The model under review builds one solid part; all positions refer to its coordinate system, in mm. Round coordinates to 2 decimals unless told otherwise and drop trailing zeros. Order: outer loops, then holes, each group sorted by start corner. A loop starts at its lowest first (then second) coordinate and runs counter-clockwise, first axis right, second up.
from build123d import *

# Parameters (mm, degrees)
SKETCH2_R           = 2.50063
SKETCH2_R_2         = 3.5687
BOSS_EXTRUDE1_DEPTH = 4.7625


with BuildPart() as part:
    # Sketch2 → Boss-Extrude1 (new body)
    with BuildSketch(Plane.XY):
        with BuildLine():
            Line((20.204627806, -155.317842979), (66.653485088, -155.317842979))
            ThreePointArc((66.653485088, -155.317842979), (69.031331892, -154.332906584), (70.016268288, -151.95505978))
            Line((70.016268288, -151.95505978), (70.009462537, -134.779191139))
            ThreePointArc((70.009462537, -134.779191139), (69.330107736, -131.296239945), (67.723101309, -128.132381176))
            Line((67.723101309, -128.132381176), (58.368571144, -114.709141578))
            ThreePointArc((58.368571144, -114.709141578), (58.101227711, -114.164618042), (58.009428426, -113.56499209))
            Line((58.009428426, -113.56499209), (58.017340801, -89.273956224))
            ThreePointArc((58.017340801, -89.273956224), (58.109330305, -88.675027543), (58.376464494, -88.131136967))
            Line((58.376464494, -88.131136967), (67.309788153, -75.311850981))
            ThreePointArc((67.309788153, -75.311850981), (69.324850125, -71.208346949), (70.017816939, -66.689606297))
            Line((70.017816939, -66.689606297), (70.017970953, -58.209892985))
            ThreePointArc((70.017970953, -58.209892985), (67.203843889, -51.415989261), (60.409940165, -48.601862197))
            Line((60.409940165, -48.601862197), (20.204627806, -48.601862197))
            ThreePointArc((20.204627806, -48.601862197), (19.517944941, -48.72344088), (18.914748074, -49.073395554))
            Line((18.914748074, -49.073395554), (5.555020387, -60.347728592))
            ThreePointArc((5.555020387, -60.347728592), (4.951823521, -60.697683266), (4.265140655, -60.819261949))
            Line((4.265140655, -60.819261949), (-4.272604079, -60.819261949))
            ThreePointArc((-4.272604079, -60.819261949), (-4.959286944, -60.697683266), (-5.562483811, -60.347728592))
            Line((-5.562483811, -60.347728592), (-18.922211498, -49.073395554))
            ThreePointArc((-18.922211498, -49.073395554), (-19.525408364, -48.72344088), (-20.212091229, -48.601862197))
            Line((-20.212091229, -48.601862197), (-60.417403588, -48.601862197))
            ThreePointArc((-60.417403588, -48.601862197), (-67.211307313, -51.415989261), (-70.025434377, -58.209892985))
            Line((-70.025434377, -58.209892985), (-70.025280362, -66.689606297))
            ThreePointArc((-70.025280362, -66.689606297), (-69.332313549, -71.208346949), (-67.317251577, -75.311850981))
            Line((-67.317251577, -75.311850981), (-58.383927917, -88.131136967))
            ThreePointArc((-58.383927917, -88.131136967), (-58.116793729, -88.675027543), (-58.024804225, -89.273956224))
            Line((-58.024804225, -89.273956224), (-58.01689185, -113.56499209))
            ThreePointArc((-58.01689185, -113.56499209), (-58.108691135, -114.164618042), (-58.376034568, -114.709141578))
            Line((-58.376034568, -114.709141578), (-67.730564733, -128.132381176))
            ThreePointArc((-67.730564733, -128.132381176), (-69.337571159, -131.296239945), (-70.016925961, -134.779191139))
            Line((-70.016925961, -134.779191139), (-70.023731711, -151.95505978))
            ThreePointArc((-70.023731711, -151.95505978), (-69.038795316, -154.332906584), (-66.660948512, -155.317842979))
            Line((-66.660948512, -155.317842979), (-20.212091229, -155.317842979))
            ThreePointArc((-20.212091229, -155.317842979), (-19.525408364, -155.196264296), (-18.922211498, -154.846309622))
            Line((-18.922211498, -154.846309622), (-5.562483811, -143.571976584))
            ThreePointArc((-5.562483811, -143.571976584), (-4.959286944, -143.22202191), (-4.272604079, -143.100443227))
            Line((-4.272604079, -143.100443227), (4.265140655, -143.100443227))
            ThreePointArc((4.265140655, -143.100443227), (4.951823521, -143.22202191), (5.555020387, -143.571976584))
            Line((5.555020387, -143.571976584), (18.914748074, -154.846309622))
            ThreePointArc((18.914748074, -154.846309622), (19.517944941, -155.196264296), (20.204627806, -155.317842979))
        make_face()
        with Locations(Location((-56.926856711, -62.252536918, 0), (0, 0, 180))):
            Circle(SKETCH2_R, mode=Mode.SUBTRACT)
        with Locations(Location((-31.926856712, -62.252536918, 0), (0, 0, 180))):
            Circle(SKETCH2_R, mode=Mode.SUBTRACT)
        with Locations(Location((31.919393288, -62.252536918, 0), (0, 0, 180))):
            Circle(SKETCH2_R, mode=Mode.SUBTRACT)
        with Locations(Location((56.919393288, -62.252536918, 0), (0, 0, 180))):
            Circle(SKETCH2_R, mode=Mode.SUBTRACT)
        with Locations(Location((-39.920054199, -81.992843779, 0), (0, 0, 180))):
            Circle(SKETCH2_R, mode=Mode.SUBTRACT)
        with Locations(Location((-39.907032742, -91.992843779, 0), (0, 0, 180))):
            Circle(SKETCH2_R, mode=Mode.SUBTRACT)
        with Locations(Location((-39.920054199, -112.317382635, 0), (0, 0, 180))):
            Circle(SKETCH2_R, mode=Mode.SUBTRACT)
        with Locations(Location((-39.907032742, -132.632843676, 0), (0, 0, 180))):
            Circle(SKETCH2_R, mode=Mode.SUBTRACT)
        with Locations(Location((-39.920054199, -142.632843676, 0), (0, 0, 180))):
            Circle(SKETCH2_R, mode=Mode.SUBTRACT)
        with Locations(Location((10.02542097, -101.992843779, 0), (0, 0, 180))):
            Circle(SKETCH2_R, mode=Mode.SUBTRACT)
        with Locations(Location((-9.97457903, -101.992843779, 0), (0, 0, 180))):
            Circle(SKETCH2_R, mode=Mode.SUBTRACT)
        with Locations(Location((39.700429549, -91.992843779, 0), (0, 0, 180))):
            Circle(SKETCH2_R, mode=Mode.SUBTRACT)
        with Locations(Location((39.700429549, -132.632843676, 0), (0, 0, 180))):
            Circle(SKETCH2_R, mode=Mode.SUBTRACT)
        with Locations(Location((-56.895356292, -141.122536917, 0), (0, 0, 180))):
            Circle(SKETCH2_R_2, mode=Mode.SUBTRACT)
        with Locations(Location((39.700429549, -142.632843676, 0), (0, 0, 180))):
            Circle(SKETCH2_R_2, mode=Mode.SUBTRACT)
        with Locations(Location((39.700429549, -112.317382635, 0), (0, 0, 180))):
            Circle(SKETCH2_R_2, mode=Mode.SUBTRACT)
        with Locations(Location((39.700429549, -81.992843779, 0), (0, 0, 180))):
            Circle(SKETCH2_R_2, mode=Mode.SUBTRACT)
        with Locations(Location((56.887892868, -141.122536917, 0), (0, 0, 180))):
            Circle(SKETCH2_R_2, mode=Mode.SUBTRACT)
    extrude(amount=BOSS_EXTRUDE1_DEPTH)


solid = part.part
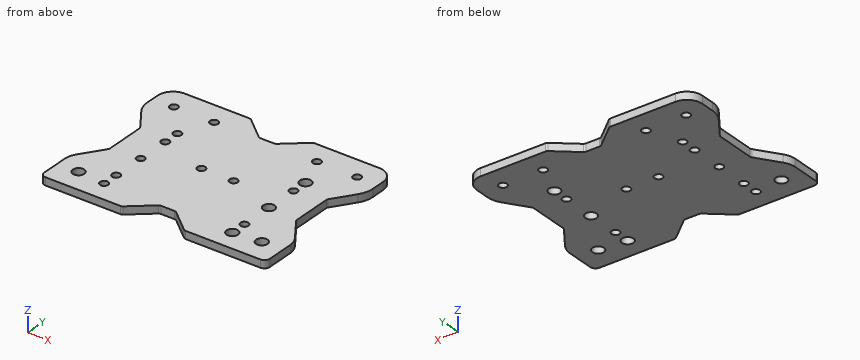
(1) Clearance check with flat-ended pins moving along their axes: P1, Ø4.5, axis at x = -9.97, y = -101.99, coming from the +Z side (3 decimals); P2, Ø1.4, axis at y = -100.5, z = 3, coming from the +X side; P3, Ø1.4, axis at y = -146, z = 3.5, coming from the +X side; P4, Ø1.5, axis at x = -13, z = 1, coming from the +Y side. State where each tip first meets the part, or that it passes through.
(2) We need section A-A (x = -39.5). Give the boundary of the cut face in (y, z).
(3) To check wall thickness, follow L1, parallel to X at y = -62, z = 4.1; L2, parallel to Y at x = 31.5, z = 0.4; L3, parallel to Y at x = 60, z = 1.3. State the ranges of each line that lie inside material, in increasing order.
(4) We need section B-B (y = -107). Give the boundary of the cut face in (x, z), and give its area (3 significant figures).
(5) We need section D-D (y = -120). Give the boundary of the cut face in (x, z), and give its area (3 significant figures).
(6) We need section C-C (z = 3.85). Count the separate pieces of the cut face and the enclosed holes in it, and give its area (3 significant figures).
Verdict:
1. P1: passes through
1. P2: stops at x = 58.01
1. P3: stops at x = 70.01
1. P4: stops at y = -53.44
2. outline: (-155.32, 0) - (-145.1, 0) - (-145.1, 4.76) - (-155.32, 4.76) - close; (-140.17, 0) - (-135.1, 0) - (-135.1, 4.76) - (-140.17, 4.76) - close; (-130.17, 0) - (-114.78, 0) - (-114.78, 4.76) - (-130.17, 4.76) - close; (-109.85, 0) - (-94.46, 0) - (-94.46, 4.76) - (-109.85, 4.76) - close; (-89.53, 0) - (-84.46, 0) - (-84.46, 4.76) - (-89.53, 4.76) - close; (-79.53, 0) - (-48.6, 0) - (-48.6, 4.76) - (-79.53, 4.76) - close
3. L1: x = -70.03 to -59.41, -54.44 to -34.41, -29.44 to 29.43, 34.41 to 54.43, 59.41 to 70.02
3. L2: y = -155.32 to -64.72, -59.79 to -48.6
3. L3: y = -155.32 to -142.87, -139.38 to -117.05, -85.8 to -48.6
4. outline: (-58.02, 0) - (58.01, 0) - (58.01, 4.76) - (-58.02, 4.76) - close
4. area: 553 mm2
5. outline: (-62.06, 0) - (62.06, 0) - (62.06, 4.76) - (-62.06, 4.76) - close
5. area: 591 mm2
6. separate pieces: 1
6. enclosed holes: 18
6. area: 12,800 mm2
